Autodesk Inventor part; units mm, degrees
ref_plane "XZ Plane" through (0, 0, 0) normal (0, 1, 0) x (-1, 0, 0)
ref_plane "XY Plane" through (0, 0, 0) normal (0, 0, 1) x (1, 0, 0)
sketch "Boceto1" plane through (0, 0, 0) normal (1, 0, 0) x (0, 1, 0)
  circle A0 centre (0, 0) radius 97.5
  dimension "d0" = 195
extrude "Extrusión1" add sketch "Boceto1" against normal blind 40
fillet "Empalme1" radius 5 2 edges at (-40, -97.5, 0) (0, -97.5, 0)
sketch "Boceto2" plane through (-40, 0, 0) normal (-1, 0, 0) x (0, 0, 1)
  circle A0 centre (0, 0) radius 10.25
  dimension "d4" = 20.5
extrude "Extrusión2" cut sketch "Boceto2" against normal up to surface (40 mm away)
properties part number "wheel_right_link"
Could you check a few things on this model? Use its own coordinates, in mm. Round coordinates to 2 decimals unless told otherwise and drop trailing zeros. Loops run counter-clockwise (first coordinate to the right, second up) from the corner with the lowest first, then second, coordinate; pieces in that order, holes last.
Q1. For P1, Ø2, axis at x = -24, z = -77, coming from the -Y side; P2, Ø10, axis at x = -7.5, z = 66.5, coming from the -Y side; P3, Ø1, axis at y = 30, z = 65, coming from the +X side; P4, Ø3, axis at x = -17, y = 60.5, coming from the -Z side, each with a flat end and sliding along its axis, tell me the tip position at first contact or that it passes through.
Q2. I want a section at A-A (z = 0). Write out the boundary of the cut face in (x, y).
Q3. I want a section at C-C (x = -17.5). Write out the boundary of the cut face in (y, z).
Q4. Thinking about a two-plate mould opening in Z: for faces 1 (the cylindrical face through (-19.79, -77.37, -59.33)), 2 (the cylindrical face through (-20.28, -10.006, -2.222)), 3 (the flat face through (-40, -1, -19)), which applies, pulls with the +Z half, pulls with the -Z half, needs draft (parallel to the pull), parting line crosses it, or undercut?
Q5. Please list where these lines run through material, in increasing order: L1, parallel to Z at x = -27, y = 2; L2, parallel to Y at x = -3.5, z = 36; L3, parallel to Y at x = -15.5, z = -80.
Answer below:
1. P1: stops at y = -61.08
1. P2: stops at y = -75.66
1. P3: stops at x = 0
1. P4: stops at z = -77.62
2. outline: (-40, -92.5) arc R5 ccw to (-35, -97.5) - (-5, -97.5) arc R5 ccw to (0, -92.5) - (0, -10.25) - (-40, -10.25) - close; (-40, 10.25) - (0, 10.25) - (0, 92.5) arc R5 ccw to (-5, 97.5) - (-35, 97.5) arc R5 ccw to (-40, 92.5) - close
3. outline: circle Ø195 at (0, 0); hole circle Ø20.5 at (0, 0)
4. face 1: parting line crosses it
4. face 2: undercut
4. face 3: needs draft
5. L1: z = -97.48 to -10.05, 10.05 to 97.48
5. L2: y = -90.36 to 90.36
5. L3: y = -55.73 to 55.73
